Verification items for this drawing (mm, ordinates from the low corner). A direction names the side the tool comes from. Give positions to 0.01 mm unless a question says otherwise; leave off trailing zeros. Write each loop counter-clockwise with the first axis right and the second up, starting at its lowest first coordinate (ties: lowest second). Pieces come first, ordered by that corner, then holes. Notation, with made-up numbers: (55, -16) -> (91, -16) arc R13 ccw to (91, -11) -> close; hole circle Ø4 at (-38.5, 16.5). An arc over 180 degrees is marked (long way). Use one line per item in the form item = value. Start each with the question number.
(1) Section check B-B, the plane x = 97. Record the cut outline in (y, z).
(2) Scan lines: L1, parallel to Z at x = 52, y = 10.25; L2, parallel to Z at x = 25, y = 24.5 (3 decimals); L3, parallel to Y at x = 67.5, z = 6. Record each from-to range of solid material in increasing order.
(3) Set-up check for the marked faces 4, 5, 6 and 7: record each of +Z, -Z, +X, -X, +Y, -Y from which the full face is reachable in a straight line by a thin tool's end or side.
(4) Section check C-C, the plane z = 77. Record the cut outline in (x, y), plus the area to 3 significant figures.
(5) Release check for a two-part mould opening along Z. For the marked faces 1, 2 and 3 record: pulls with the +Z half, pulls with the -Z half, needs draft (parallel to the pull), parting line crosses it, or undercut.
(6) Depth check by flat-ended pin: pin 1 Ø8.5 at (x, z) = (30.5, 68) entering from +Y; pin 2 Ø6 at (y, z) = (12.5, 71) entering from -X; pin 3 Ø19.5 at (x, z) = (91.5, 10.5) entering from -Y; pin 4 Ø3 at (y, z) = (9, 71) entering from -X. Enter the tip coordinate at first touch or a pass-through.
(7) Section check A-A, the plane y = 23.75. Record the cut outline in (x, z) (3 decimals), plus the area to 3 significant figures.
(8) Section check D-D, the plane x = 57.5. Record the cut outline in (y, z) (3 decimals), plus the area to 3 significant figures.
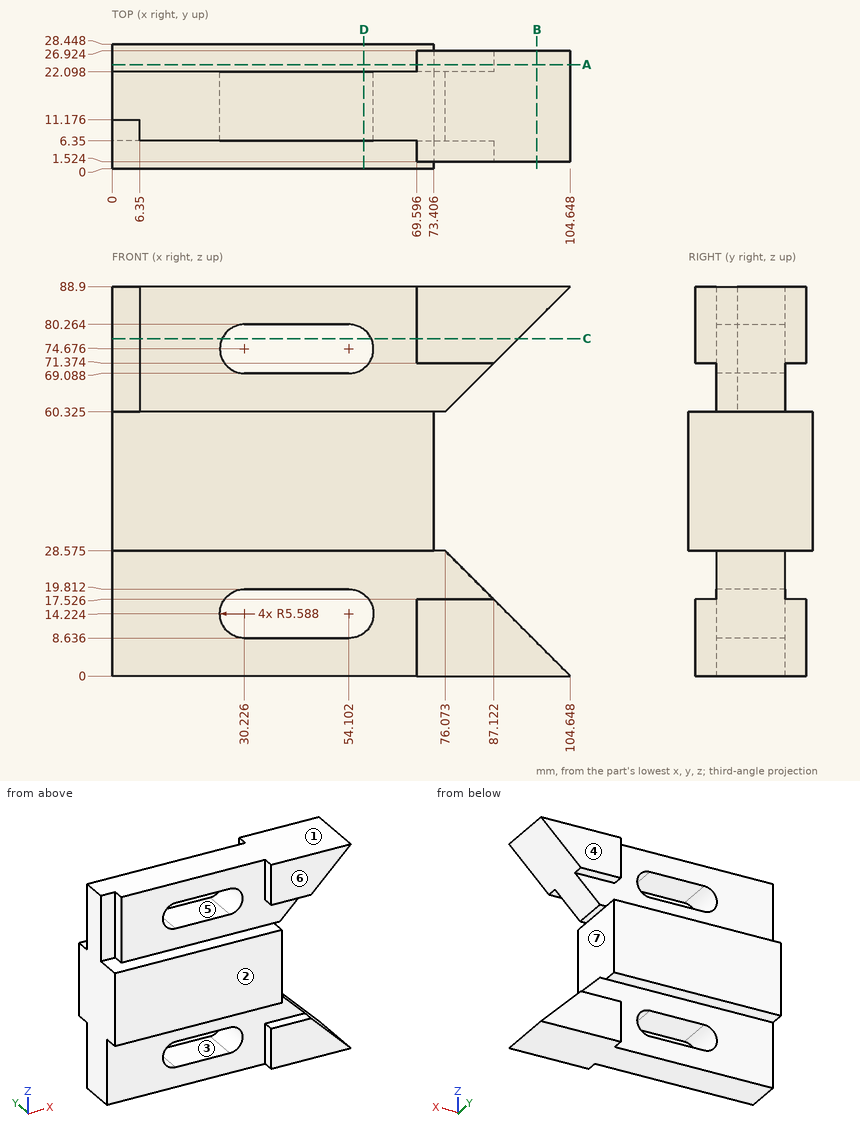
Completed:
q1.outline = (1.52, 0) -> (26.92, 0) -> (26.92, 7.65) -> (1.52, 7.65) -> close; (1.52, 81.25) -> (26.92, 81.25) -> (26.92, 88.9) -> (1.52, 88.9) -> close
q2.L1 = 0 to 8.64, 19.81 to 69.09, 80.26 to 88.9
q2.L2 = 28.575 to 60.325
q2.L3 = 6.35 to 22.1
q3.face_4 = +Z, +X, -X, +Y
q3.face_5 = +Y, -Y
q3.face_6 = +Z, +X, -X, -Y
q3.face_7 = +X, +Y, -Y
q4.outline = (0, 11.18) -> (6.35, 11.18) -> (6.35, 6.35) -> (25.14, 6.35) -> (25.14, 22.1) -> (0, 22.1) -> close; (59.18, 6.35) -> (69.6, 6.35) -> (69.6, 1.52) -> (92.75, 1.52) -> (92.75, 26.92) -> (69.6, 26.92) -> (69.6, 22.1) -> (59.18, 22.1) -> close
q4.area = 1,120 mm²
q5.face_1 = pulls with the +Z half
q5.face_2 = needs draft
q5.face_3 = undercut
q6.pin_1 = 22.1
q6.pin_2 = 0
q6.pin_3 = 1.52
q6.pin_4 = 6.35
q7.outline = (0, 28.575) -> (73.406, 28.575) -> (73.406, 60.325) -> (0, 60.325) -> close; (69.596, 0) -> (104.648, 0) -> (87.122, 17.526) -> (69.596, 17.526) -> close; (69.596, 71.374) -> (87.122, 71.374) -> (104.648, 88.9) -> (69.596, 88.9) -> close
q7.area = 3,250 mm²
q8.outline = (0, 28.575) -> (6.35, 28.575) -> (6.35, 18.66) -> (22.098, 18.66) -> (22.098, 28.575) -> (28.448, 28.575) -> (28.448, 60.325) -> (22.098, 60.325) -> (22.098, 70.24) -> (6.35, 70.24) -> (6.35, 60.325) -> (0, 60.325) -> close; (6.35, 0) -> (22.098, 0) -> (22.098, 9.788) -> (6.35, 9.788) -> close; (6.35, 79.112) -> (22.098, 79.112) -> (22.098, 88.9) -> (6.35, 88.9) -> close
q8.area = 1,520 mm²
